from build123d import *

# Parameters (mm, degrees)
EXTRUDE_1_DEPTH     = 6
SKETCH_2_R          = 3
EXTRUDE_2_DEPTH     = 1.5
SKETCH_3_R          = 3
EXTRUDE_3_DEPTH     = 1.5
SKETCH_4_R          = 2
EXTRUDE_4_DEPTH     = 2
SKETCH_5_R          = 2.1
EXTRUDE_5_DEPTH     = 1
CHAMFER_1_SIZE      = 0.2
SKETCH_6_W          = 1
SKETCH_6_H          = 5
CUT_EXTRUDE_1_DEPTH = 2
SKETCH_7_R          = 2
EXTRUDE_6_DEPTH     = 7.5
CHAMFER_2_SIZE      = 0.2


with BuildPart() as part:
    # 草图1 → 凸台-拉伸1 (new body)
    with BuildSketch(Plane.XY):
        Polygon((0, 0), (11, 0), (14, -6), (18.5, -6), (18.5, -7.5), (13.072949017, -7.5), (10.072949017, -1.5), (0, -1.5), align=None)
    extrude(amount=EXTRUDE_1_DEPTH)

    # 草图2 → 凸台-拉伸2 (add)
    with BuildSketch(Plane(origin=(0, 0, 0), x_dir=(1, 0, 0), z_dir=(0, 1, 0))):
        with Locations((0, -3)):
            Circle(SKETCH_2_R)
    extrude(amount=-EXTRUDE_2_DEPTH)

    # 草图3 → 凸台-拉伸3 (add)
    with BuildSketch(Plane(origin=(0, -6, 0), x_dir=(1, 0, 0), z_dir=(0, 1, 0))):
        with Locations((18.5, -3)):
            Circle(SKETCH_3_R)
    extrude(amount=-EXTRUDE_3_DEPTH)

    # 草图4 → 凸台-拉伸4 (add)
    with BuildSketch(Plane.XZ.offset(1.5)):
        with Locations(Location((0, 3, 0), (0, 0, 90))):
            Circle(SKETCH_4_R)
    extrude(amount=EXTRUDE_4_DEPTH)

    # 草图5 → 凸台-拉伸5 (add)
    with BuildSketch(Plane.XZ.offset(3.5)):
        with Locations(Location((0, 3, 0), (0, 0, 270))):
            Circle(SKETCH_5_R)
    extrude(amount=EXTRUDE_5_DEPTH)

    # 倒角1
    chamfer_1_edges = [part.edges().sort_by_distance(p)[0] for p in [
        (0, -4.5, 5.1),
    ]]
    chamfer(chamfer_1_edges, length=CHAMFER_1_SIZE)

    # 草图6 → 切除-拉伸1 (cut)
    with BuildSketch(Plane.XZ.offset(4.5)):
        with Locations((0, 3)):
            Rectangle(SKETCH_6_W, SKETCH_6_H)
    extrude(amount=-CUT_EXTRUDE_1_DEPTH, mode=Mode.SUBTRACT)

    # 草图7 → 凸台-拉伸6 (add)
    with BuildSketch(Plane(origin=(0, -6, 0), x_dir=(1, 0, 0), z_dir=(0, 1, 0))):
        with Locations((18.5, -3)):
            Circle(SKETCH_7_R)
    extrude(amount=EXTRUDE_6_DEPTH)

    # 倒角2
    chamfer_2_edges = [part.edges().sort_by_distance(p)[0] for p in [
        (16.5, 1.5, 3),
    ]]
    chamfer(chamfer_2_edges, length=CHAMFER_2_SIZE)


solid = part.part
Verification items for the finished model (mm, model axes). A direction names the side the tool comes from. Give positions to 0.01 mm unless a question says otherwise; leave off trailing zeros. Write each loop counter-clockwise with the first axis right and the second up, starting at its lowest first coordinate (ties: lowest second). Pieces come first, ordered by that corner, then holes.
(1) Access from +Z, -Z, +X, -X, +Y, -Y to the whole of each face (thin tool, end or side, straight path). Record for faces 5 (the face through (16, -6, 3)), 6 (the face through (11.594, -4.542, 2.958)), 7 (the face through (12.5, -3, 3)).
(2) Cross-section at B-B (z = 3). Enter the section's corners in (x, y), plus the area to 3 significant figures.
(3) Cross-section at D-D (y = 0.75). Enter the section's corners in (x, z), plus the area to 3 significant figures.
(4) Gauge pin test, flat ends, axial feed: pin 1 (2 mm diameter, centred on x = 8, z = 4, fed in from -Y); pin 2 (2 mm diameter, centred on y = -3, z = 3.5, fed in from -X); pin 3 (0.8 mm diameter, centred on x = 0, z = 3, fed in from -Y). Record the tip position at first contact, or that the pin passes through.
(5) Mould release check, pull along X, two halves, no side actions. Record for faces 1 (the face through (2.1, -3.9, 3)), 2 (the face through (21.5, -6.7, 3.1)), 3 (the face through (1, -4.5, 3)), 4 (the face through (0.766, -2.486, 4.847)): +X half, -X half, draft (parallel to the pull), parting line (faces both ways), or undercut.
(6) Cross-section at C-C (x = 15). Enter the section's corners in (y, z), plus the area to 3 significant figures.
(7) Cross-section at A-A (y = -3.25). Enter the section's corners in (x, z) (1 decimal).
(8) Material ranges on line 1 (Y direction, x = 6, z = 1.3); line 2 (Y direction, x = 0.75, z = 3.2); line 3 (X direction, y = -5.5, z = 1.3), recorded low to high.
Worked out:
1. face 5: +Y
1. face 6: +Z, -Z, -Y
1. face 7: +Z, -Z, +Y
2. outline: (-3, -1.5) - (-2, -1.5) - (-2, -3.5) - (-2.1, -3.5) - (-2.1, -4.3) - (-1.9, -4.5) - (-0.5, -4.5) - (-0.5, -2.5) - (0.5, -2.5) - (0.5, -4.5) - (1.9, -4.5) - (2.1, -4.3) - (2.1, -3.5) - (2, -3.5) - (2, -1.5) - (10.07, -1.5) - (13.07, -7.5) - (21.5, -7.5) - (21.5, -6) - (20.5, -6) - (20.5, 1.3) - (20.3, 1.5) - (16.7, 1.5) - (16.5, 1.3) - (16.5, -6) - (14, -6) - (11, 0) - (-3, 0) - close
2. area: 82.4 mm2
3. outline: circle Ø4 at (18.5, 3)
3. area: 12.6 mm2
4. pin 1: stops at y = -1.5
4. pin 2: stops at x = -2.1
4. pin 3: stops at y = -2.5
5. face 1: undercut
5. face 2: +X half
5. face 3: draft
5. face 4: undercut
6. outline: (-7.5, 0) - (-6, 0) - (-6, 6) - (-7.5, 6) - close
6. area: 9.00 mm2
7. outline: (-0.5, 1.1) - (-0.5, 4.9) arc R2 ccw to start; (0.5, 1.1) arc R2 ccw to (0.5, 4.9) - close; (10.9, 0) - (12.6, 0) - (12.6, 6) - (10.9, 6) - close; circle Ø4 at (18.5, 3)
8. line 1: y = -1.5 to 0
8. line 2: y = -4.5 to 0
8. line 3: x = 12.07 to 13.75, 17.45 to 19.55
